Verification items for the finished model (mm, model axes). A direction names the side the tool comes from. Coordinates: 2 decimals unless noted, no trailing zeros. Write each loop counter-clockwise with the first axis right and the second up, starting at its lowest first coordinate (ties: lowest second). Pieces come first, ordered by that corner, then holes. Notation, with made-up numbers: M -5.75,71 L 5.25,71 A10 ccw 5.25,76 Z; hole C -34,2 d3. An arc over 180 degrees is marked long. Answer in a Markdown table with one row per item.
from build123d import *

# Parameters (mm, degrees)
SKETCH1_W           = 34
SKETCH1_H           = 15.8
BOSS_EXTRUDE1_DEPTH = 3
BOSS_EXTRUDE2_DEPTH = 8
CUT_EXTRUDE1_DEPTH  = 99.217047801
SKETCH4_R           = 2
BOSS_EXTRUDE3_DEPTH = 3
FILLET1_R           = 1
SKETCH5_R           = 1.5
CUT_EXTRUDE2_DEPTH  = 99.506794074
CUT_EXTRUDE3_DEPTH  = 3


with BuildPart() as part:
    # Sketch1 → Boss-Extrude1 (new body)
    with BuildSketch(Plane.XY):
        with Locations((71.801699099, 33.292799322)):
            Rectangle(SKETCH1_W, SKETCH1_H)
    extrude(amount=BOSS_EXTRUDE1_DEPTH)

    # Sketch2 → Boss-Extrude2 (add)
    with BuildSketch(Plane.XY.offset(3)):
        with BuildLine():
            Line((63.551699099, 37.792799322), (77.051699099, 37.792799322))
            ThreePointArc((77.051699099, 37.792799322), (79.173019442, 36.914119666), (80.051699099, 34.792799322))
            Line((80.051699099, 34.792799322), (80.051699099, 31.792799322))
            ThreePointArc((80.051699099, 31.792799322), (79.173019442, 29.671478979), (77.051699099, 28.792799322))
            Line((77.051699099, 28.792799322), (63.551699099, 28.792799322))
            Line((63.551699099, 28.792799322), (63.551699099, 37.792799322))
        make_face()
    extrude(amount=BOSS_EXTRUDE2_DEPTH)

    # Sketch3 → Cut-Extrude1 (cut, through all)
    with BuildSketch(Plane.XY.offset(3)):
        Polygon((54.801699099, 41.192799322), (62.801699099, 41.192799322), (61.121201007, 38.792799322), (54.801699099, 38.792799322), align=None)
        Polygon((62.801699099, 25.392799322), (61.121201007, 27.792799322), (54.801699099, 27.792799322), (54.801699099, 25.392799322), align=None)
        Polygon((88.801699099, 25.392799322), (80.801699099, 25.392799322), (82.48219719, 27.792799322), (88.801699099, 27.792799322), align=None)
        Polygon((80.801699099, 41.192799322), (82.48219719, 38.792799322), (88.801699099, 38.792799322), (88.801699099, 41.192799322), align=None)
    extrude(amount=-CUT_EXTRUDE1_DEPTH, mode=Mode.SUBTRACT)

    # Sketch4 → Boss-Extrude3 (add)
    with BuildSketch(Plane.XY.offset(11)):
        with Locations((67.051699099, 33.292799322)):
            Circle(SKETCH4_R)
        with Locations((76.551699099, 33.292799322)):
            Circle(SKETCH4_R)
    extrude(amount=BOSS_EXTRUDE3_DEPTH)

    # Fillet1
    fillet1_edges = [part.edges().sort_by_distance(p)[0] for p in [
        (80.801699099, 41.192799322, 1.5),
        (88.801699099, 38.792799322, 1.5),
        (82.48219719, 38.792799322, 1.5),
        (88.801699099, 27.792799322, 1.5),
        (80.801699099, 25.392799322, 1.5),
        (82.48219719, 27.792799322, 1.5),
        (62.801699099, 25.392799322, 1.5),
        (54.801699099, 27.792799322, 1.5),
        (61.121201007, 27.792799322, 1.5),
        (54.801699099, 38.792799322, 1.5),
        (62.801699099, 41.192799322, 1.5),
        (61.121201007, 38.792799322, 1.5),
    ]]
    fillet(fillet1_edges, radius=FILLET1_R)

    # Sketch5 → Cut-Extrude2 (cut, through all)
    with BuildSketch(Plane.XY.offset(3)):
        with Locations((59.301699099, 33.292799322)):
            Circle(SKETCH5_R)
        with Locations((84.301699099, 33.292799322)):
            Circle(SKETCH5_R)
    extrude(amount=-CUT_EXTRUDE2_DEPTH, mode=Mode.SUBTRACT)

    # Sketch6 → Cut-Extrude3 (cut)
    with BuildSketch(Plane(origin=(0, 0, 0), x_dir=(-1, 0, 0), z_dir=(0, 0, -1))):
        with BuildLine():
            Line((-77.801699099, 36.792799322), (-65.801699099, 36.792799322))
            ThreePointArc((-65.801699099, 36.792799322), (-64.387485536, 36.207012885), (-63.801699099, 34.792799322))
            Line((-63.801699099, 34.792799322), (-63.801699099, 31.792799322))
            ThreePointArc((-63.801699099, 31.792799322), (-64.387485536, 30.37858576), (-65.801699099, 29.792799322))
            Line((-65.801699099, 29.792799322), (-77.801699099, 29.792799322))
            ThreePointArc((-77.801699099, 29.792799322), (-79.215912661, 30.37858576), (-79.801699099, 31.792799322))
            Line((-79.801699099, 31.792799322), (-79.801699099, 34.792799322))
            ThreePointArc((-79.801699099, 34.792799322), (-79.215912661, 36.207012885), (-77.801699099, 36.792799322))
        make_face()
    extrude(amount=-CUT_EXTRUDE3_DEPTH, mode=Mode.SUBTRACT)


solid = part.part
1) Release check for a two-part mould opening along Y. For faces 4 (the face through (59.99, 31.96, 1.52)), 5 (the face through (67, 33, 14)), 6 (the face through (82.547, 27.683, 1.479)) record: +Y half, -Y half, draft (parallel to the pull), parting line (faces both ways), or undercut.
Response values:
| item | result |
|---|---|
| face 4 | undercut |
| face 5 | draft |
| face 6 | -Y half |
2) Sectioned sample at A-A (z = 1.5). Give the number of separate pieces and of enclosed holes in the cut face, then the cut area to 3 significant figures.
Response values:
| item | result |
|---|---|
| separate pieces | 1 |
| enclosed holes | 3 |
| area | 345 mm² |
3) Thickness scan on L1, parallel to Y at x = 75, z = 1; L2, parallel to X at y = 33, z = 1.25; L3, parallel to Z at x = 59.5, y = 38.25. Record the ranges inside material, lowest first. Write a range as [from, to].
Response values:
| item | result |
|---|---|
| L1 | y = [25.39, 29.79], [36.79, 41.19] |
| L2 | x = [54.8, 57.83], [60.77, 63.8], [79.8, 82.83], [85.77, 88.8] |
| L3 | z = [0, 3] |
4) Tool access check on faces 1 (the face through (72, 39, 3)), 2 (the face through (72, 33, 3)), 3 (the face through (63.552, 33, 7)). Record the directions out of +Z, -Z, +X, -X, +Y, -Y that give a thin tool (end or side, any length) a straight path to the whole face; none if there is none.
Response values:
| item | result |
|---|---|
| face 1 | +Z |
| face 2 | -Z |
| face 3 | +Z, -X, +Y, -Y |
5) Sectioned sample at D-D (y = 27). Record the cut outline in (x, z), then the cut area to 3 significant figures.
Response values:
| item | result |
|---|---|
| outline | M 61.68,0 L 81.93,0 L 81.93,3 L 61.68,3 Z |
| area | 60.8 mm² |
6) Sectioned sample at C-C (z = 8). Record the cut outline in (x, y), then the cut area to 3 significant figures.
Response values:
| item | result |
|---|---|
| outline | M 63.55,28.79 L 77.05,28.79 A3 ccw 80.05,31.79 L 80.05,34.79 A3 ccw 77.05,37.79 L 63.55,37.79 Z |
| area | 145 mm² |
7) Depth check by flat-ended pin: pin 1 (2.5 mm diameter, centred on y = 32.5, z = 6.5, fed in from +X); pin 2 (0.9 mm diameter, centred on x = 86.5, z = 2, fed in from -Y); pin 3 (1.5 mm diameter, centred on x = 74.5, z = 5.5, fed in from -Y). Enter the tip coordinate at first touch or a pass-through.
Response values:
| item | result |
|---|---|
| pin 1 | stops at x = 80.05 |
| pin 2 | stops at y = 27.79 |
| pin 3 | stops at y = 28.79 |
8) Sectioned sample at B-B (x = 87). Record the cut outline in (y, z), then the cut area to 3 significant figures.
Response values:
| item | result |
|---|---|
| outline | M 27.79,0 L 38.79,0 L 38.79,3 L 27.79,3 Z |
| area | 33.0 mm² |
